from build123d import *

# Parameters (mm, degrees)
F1_DEPTH = 5


with BuildPart() as f1:
    # F0 (on Top) → F1 (new body)
    with BuildSketch(Plane.XY):
        with BuildLine():
            Line((-27, -3), (27, -3))
            ThreePointArc((27, -3), (29.12132, -2.12132), (30, 0))
            ThreePointArc((30, 0), (29.12132, 2.12132), (27, 3))
            Line((27, 3), (-27, 3))
            ThreePointArc((-27, 3), (-29.12132, 2.12132), (-30, 0))
            ThreePointArc((-30, 0), (-29.12132, -2.12132), (-27, -3))
        make_face()
        with BuildLine():
            ThreePointArc((1.428286, 1.4), (0, -2), (-1.428286, 1.4))
            Line((-1.428286, 1.4), (1.428286, 1.4))
        make_face(mode=Mode.SUBTRACT)
    extrude(amount=F1_DEPTH)


solid = f1.part
Source: CAD feature listing. Evaluate the final solid. Frame: model axes, mm. Coordinates: 2 decimals unless noted, no trailing zeros. Loops run counter-clockwise (first coordinate to the right, second up) from the corner with the lowest first, then second, coordinate; pieces in that order, holes last. Notation, with made-up numbers: (69, 75) -> (127, 75) arc R29 ccw to (127, 100) -> close; hole circle Ø9 at (31, 56.25). An arc over 180 degrees is marked (long way). Answer in a Markdown table with one row per item. Add a question column.
Q1. Section A-A on z = 1.8. Return the cut outline in (x, y).
Q2. Pull-direction query (X, two-part tool) for faces 1 (the face through (0, 3, 2)), 2 (the face through (0, 1.4, 2)); classes: pulls with the +X half, pulls with the -X half, needs draft (parallel to the pull), parting line crosses it, or undercut.
Q3. Ray query, line 1 along Y through (x, z) = (0, 2.75); line 2 along Y through (x, z) = (1, 3.9); line 3 along X through (y, z) = (1, 3.65). Return the intervals inside material, ascending.
Q4. Section B-B on y = -0.5. Return the cut outline in (x, z), and give its area (3 significant figures).
Computed values:
| question | item | result |
|---|---|---|
| 1 | outline | (-30, 0) arc R3 ccw to (-27, -3) -> (27, -3) arc R3 ccw to (30, 0) arc R3 ccw to (27, 3) -> (-27, 3) arc R3 ccw to start; hole (-1.43, 1.4) arc R2 ccw (long way) to (1.43, 1.4) -> close |
| 2 | face 1 | needs draft |
| 2 | face 2 | undercut |
| 3 | line 1 | y = -3 to -2, 1.4 to 3 |
| 3 | line 2 | y = -3 to -1.73, 1.4 to 3 |
| 3 | line 3 | x = -29.83 to -1.73, 1.73 to 29.83 |
| 4 | outline | (-29.96, 0) -> (-1.94, 0) -> (-1.94, 5) -> (-29.96, 5) -> close; (1.94, 0) -> (29.96, 0) -> (29.96, 5) -> (1.94, 5) -> close |
| 4 | area | 280 mm^2 |
